```python
from build123d import *

# Parameters (mm, degrees)
SKETCH1_R                 = 2
BOSS_EXTRUDE1_DEPTH       = 3
SKETCH2_W                 = 1
SKETCH2_H                 = 2
CUT_EXTRUDE1_DEPTH        = 15
SKETCH3_R                 = 0.5
BOSS_EXTRUDE2_DEPTH       = 5
CUT_EXTRUDE2_DEPTH        = 5
BOSS_EXTRUDE3_DEPTH       = 3
BOSS_EXTRUDE4_DEPTH       = 2
F_1_0MM_DOWEL_HOLE1_D     = 1
F_1_0MM_DOWEL_HOLE1_DEPTH = 2
F_1_0MM_DOWEL_HOLE1_TIP   = 0.30043031


with BuildPart() as part:
    # Sketch1 → Boss-Extrude1 (new body)
    with BuildSketch(Plane.XY):
        with BuildLine():
            Line((0, 0), (11, 0))
            Line((11, 0), (11, 8))
            Line((11, 8), (6, 8))
            Line((6, 8), (6, 10))
            Line((6, 10), (0, 10))
            ThreePointArc((0, 10), (-5, 5), (0, 0))
        make_face()
        with Locations((0, 5)):
            Circle(SKETCH1_R, mode=Mode.SUBTRACT)
    extrude(amount=BOSS_EXTRUDE1_DEPTH)

    # Sketch2 → Cut-Extrude1 (cut)
    with BuildSketch(Plane(origin=(6, 0, 0), x_dir=(0, 0, -1), z_dir=(1, 0, 0))):
        with Locations((-0.5, 9)):
            Rectangle(SKETCH2_W, SKETCH2_H)
    extrude(amount=-CUT_EXTRUDE1_DEPTH, mode=Mode.SUBTRACT)

    # Sketch3 → Boss-Extrude2 (add)
    with BuildSketch(Plane.XY.offset(3)):
        Polygon((11, 8), (11, 0), (0, 0), (6, 4), (6, 8), align=None)
        with Locations((8.5, 6)):
            Circle(SKETCH3_R, mode=Mode.SUBTRACT)
    extrude(amount=BOSS_EXTRUDE2_DEPTH)

    # Sketch4 → Cut-Extrude2 (cut)
    with BuildSketch(Plane.XY.offset(8)):
        with BuildLine():
            Line((7, 8), (7, 6))
            ThreePointArc((7, 6), (8.5, 4.5), (10, 6))
            Line((10, 6), (10, 8))
            Line((10, 8), (7, 8))
        make_face()
    extrude(amount=-CUT_EXTRUDE2_DEPTH, mode=Mode.SUBTRACT)

    # Sketch5 → Boss-Extrude3 (add)
    with BuildSketch(Plane.XY.offset(3)):
        with BuildLine():
            Line((3, 2), (-4, 2))
            ThreePointArc((-4, 2), (-2.236067977, 0.527864045), (0, 0))
            Line((0, 0), (3, 2))
        make_face()
    extrude(amount=BOSS_EXTRUDE3_DEPTH)

    # Sketch6 → Boss-Extrude4 (add)
    with BuildSketch(Plane.XY.offset(3)):
        with BuildLine():
            Line((3, 10), (3, 5))
            ThreePointArc((3, 5), (2.121320344, 2.878679656), (0, 2))
            Line((0, 2), (3, 2))
            Line((3, 2), (6, 4))
            Line((6, 4), (6, 10))
            Line((6, 10), (3, 10))
        make_face()
    extrude(amount=BOSS_EXTRUDE4_DEPTH)

    # Ø1.0mm Dowel Hole1
    with Locations(Plane(origin=(8.5, 6, 3), x_dir=(1, 0, 0), z_dir=(0, 0, 1))):
        with Locations((0, 0)):
            Hole(F_1_0MM_DOWEL_HOLE1_D / 2, depth=F_1_0MM_DOWEL_HOLE1_DEPTH)
            with Locations((0, 0, -(F_1_0MM_DOWEL_HOLE1_DEPTH + F_1_0MM_DOWEL_HOLE1_TIP / 2))):  # 118° drill point
                Cone(0, F_1_0MM_DOWEL_HOLE1_D / 2, F_1_0MM_DOWEL_HOLE1_TIP, mode=Mode.SUBTRACT)


solid = part.part
```
For this review, take the finished solid that the model builds, in its own axes (mm). A direction names the side the tool comes from. Round coordinates to 2 decimals unless told otherwise and drop trailing zeros. Write each loop counter-clockwise with the first axis right and the second up, starting at its lowest first coordinate (ties: lowest second). Pieces come first, ordered by that corner, then holes. Notation, with made-up numbers: (36.25, 69) - (80.25, 69) arc R21 cw to (80.25, 96) - close; hole circle Ø6 at (-38, 31). An arc over 180 degrees is marked (long way). Put each result on its own line as item: value.
Q1. Mouldability with a two-part tool opening along Y and no side actions: class faces 6 (the face through (6, 9, 3)), 7 (the face through (2.14, 2.9, 3.99)), 8 (the face through (8, 6, 2)), 9 (the face through (8.43, 5.95, 0.75)) as released by +Y, released by -Y, zero draft, split by the parting line, or undercut.
Solved:
face 6: zero draft
face 7: released by +Y
face 8: undercut
face 9: undercut
Q2. Machinability: for faces 1 (the face through (6, 0, 4)), 2 (the face through (4, 6, 5)), 3 (the face through (8.5, 4.5, 5.5)), 4 (the face through (3, 4, 0)), 5 (the face through (1, 9, 1)), which of the approach directions +Z, -Z, +X, -X, +Y, -Y give a long, thin tool a straight path to every point of the face, cutting with its end or side? Answer none if there is none.
Solved:
face 1: +Z, -Z, +X, -X, -Y
face 2: +Z, -X, +Y
face 3: +Z, +Y
face 4: -Z, +X, -X, +Y, -Y
face 5: -Z, +X, -X, +Y
Q3. We need section D-D (y = 6.75). Give the boundary of the cut face in (x, z).
Solved:
outline: (-4.68, 0) - (-0.97, 0) - (-0.97, 3) - (-4.68, 3) - close; (0.97, 0) - (11, 0) - (11, 8) - (10, 8) - (10, 3) - (7, 3) - (7, 8) - (6, 8) - (6, 5) - (3, 5) - (3, 3) - (0.97, 3) - close
Q4. We need section A-A (z = 1.25). Give the boundary of the cut face in (x, y), and give its area (3 significant figures).
Solved:
outline: (0, 0) - (11, 0) - (11, 8) - (6, 8) - (6, 10) - (0, 10) arc R5 ccw to start; hole circle Ø4 at (0, 5); hole circle Ø1 at (8.5, 6)
area: 126 mm2
Q5. Wall thickness on probe 1 along Y at (x, z) = (0, 0.6); probe 2 along X at (y, z) = (6, 6.25); probe 3 along Y at (x, z) = (0, 1.25): over which ranges is each line inside the solid? List them lowest first.
Solved:
probe 1: y = 0 to 3, 7 to 8
probe 2: x = 6 to 7, 10 to 11
probe 3: y = 0 to 3, 7 to 10
Q6. We need section C-C (z = 4.5). Give the boundary of the cut face in (x, y).
Solved:
outline: (-4, 2) arc R5 ccw to (0, 0) - (11, 0) - (11, 8) - (10, 8) - (10, 6) arc R1.5 cw to (7, 6) - (7, 8) - (6, 8) - (6, 10) - (3, 10) - (3, 5) arc R3 cw to (0, 2) - close
Q7. Insertion check: pin 1 Ø0.9 at (y, z) = (5.5, 6) entering from -X; pin 2 Ø1.6 at (y, z) = (6.5, 5) entering from -X; pin 3 Ø3 at (x, y) = (3.5, 4) entering from -Z; pin 4 Ø1 at (y, z) = (9.5, 2) entering from +X. Each pin has a flat end and moves straight along its axis. Give the tip position at first contact, or say it passes through.
Solved:
pin 1: stops at x = 6
pin 2: stops at x = 3
pin 3: stops at z = 0
pin 4: stops at x = 6
